Here's how the part is built. I have some questions about the finished solid (model axes, mm). A direction names the side the tool comes from. Give positions to 0.01 mm unless a question says otherwise; leave off trailing zeros. Loops run counter-clockwise (first coordinate to the right, second up) from the corner with the lowest first, then second, coordinate; pieces in that order, holes last.
Q1. If we section it at D-D (z = -39): Please give me the cut outline in (x, y), plus the area to 4 significant figures.
Q2. If we section it at A-A (x = 90): Please give me the cut outline in (y, z).
Q3. For faces 1 (the face through (90, 1, -8.2)), 2 (the face through (66, 3, -25)), which set-ups out of +Z, -Z, +X, -X, +Y, -Y let a thin tool reach every point of the face, with its end or its side?
Q4. If we section it at B-B (y = 2): Please give me the cut outline in (x, z), plus the area to 3 significant figures.
Q5. I need wall thicknesses on line 1 (X direction, y = 2.85, z = -16.5); line 2 (Z direction, x = 36, y = 2.65); line 3 (Z direction, x = 64.75, y = 1.2). Which ranges of each line are inside material? Lowest first, please.
Q6. We'd pull the mould along X, two halves only. Please class faces 3 (the face through (64, 1, 0)), 4 (the face through (39, 1, -29.2)), 5 (the face through (0, 1, -26)), 6 (the face through (129.5, 1, -25)): +X half, -X half, draft (parallel to the pull), parting line (faces both ways), or undercut.
Q7. If we section it at C-C (z = -16): Please give me the cut outline in (x, y).
Autodesk Inventor part; units mm, degrees
ref_plane "YZ Plane" through (0, 0, 0) normal (1, 0, 0) x (0, 1, 0)
ref_plane "XZ Plane" through (0, 0, 0) normal (0, 1, 0) x (-1, 0, 0)
ref_plane "XY Plane" through (0, 0, 0) normal (0, 0, 1) x (1, 0, 0)
sketch "Skizze1" plane through (0, 0, 0) normal (0, 1, 0) x (-1, 0, 0)
  line L0 (0, 0) -> (-129.5, 0)
  line L1 (-129.5, 0) -> (-129.5, -51.5)
  line L2 (-129.5, -51.5) -> (0, -51.5)
  line L3 (0, -51.5) -> (0, 0)
  line L4 (-29.65, -29.2) -> (-48.65, -29.2)
  line L5 (-48.65, -29.2) -> (-48.65, -8.2)
  line L6 (-48.65, -8.2) -> (-29.65, -8.2)
  line L7 (-29.65, -8.2) -> (-29.65, -29.2)
  line L8 (-80.85, -29.2) -> (-99.85, -29.2)
  line L9 (-99.85, -29.2) -> (-99.85, -8.2)
  line L10 (-99.85, -8.2) -> (-80.85, -8.2)
  line L11 (-80.85, -8.2) -> (-80.85, -29.2)
  line L12 (-48.65, -18.7) -> (-80.85, -18.7) construction
  circle A0 centre (-64.75, -39) radius 3.5
  line L13 (-64.75, -42.5) -> (-64.75, -51.5) construction
  point P0 (-64.75, -18.7)
  point P1 (0, -25.75)
  dimension "d10" = 7
  dimension "d0" = 129.5
  dimension "d4" = 19
  dimension "d5" = 21
  dimension "d7" = 8.2
  dimension "d8" = 51.5
  dimension "d9" = 32.2
  dimension "d11" = 9
extrude "Extrusion1" add sketch "Skizze1" along normal blind 3
properties part number "wood_front"
Check sheet entries:
1. outline: (0, 0) - (61.25, 0) - (61.25, 3) - (0, 3) - close; (68.25, 0) - (129.5, 0) - (129.5, 3) - (68.25, 3) - close
1. area: 367.5 mm2
2. outline: (0, -51.5) - (3, -51.5) - (3, -29.2) - (0, -29.2) - close; (0, -8.2) - (3, -8.2) - (3, 0) - (0, 0) - close
3. face 1: +Y, -Y
3. face 2: +Z, -Z, +X, -X, +Y
4. outline: (0, -51.5) - (129.5, -51.5) - (129.5, 0) - (0, 0) - close; hole (29.65, -29.2) - (48.65, -29.2) - (48.65, -8.2) - (29.65, -8.2) - close; hole circle Ø7 at (64.75, -39); hole (80.85, -29.2) - (99.85, -29.2) - (99.85, -8.2) - (80.85, -8.2) - close
4. area: 5,830 mm2
5. line 1: x = 0 to 29.65, 48.65 to 80.85, 99.85 to 129.5
5. line 2: z = -51.5 to -29.2, -8.2 to 0
5. line 3: z = -51.5 to -42.5, -35.5 to 0
6. face 3: draft
6. face 4: undercut
6. face 5: -X half
6. face 6: +X half
7. outline: (0, 0) - (29.65, 0) - (29.65, 3) - (0, 3) - close; (48.65, 0) - (80.85, 0) - (80.85, 3) - (48.65, 3) - close; (99.85, 0) - (129.5, 0) - (129.5, 3) - (99.85, 3) - close
